Can you work these out from the model? Positions are in its coordinate system, mm. Face numbers are marked on the shaded views. A direction names the side the tool comes from. Round coordinates to 2 decimals unless told otherwise and drop trailing zeros. Loops run counter-clockwise (first coordinate to the right, second up) from the corner with the lowest first, then second, coordinate; pieces in that order, holes last.
from build123d import *

# Parameters (mm, degrees)
F1_DEPTH = 40
F2_R     = 19.99999
F3_F1_R  = 5
F3_F2_R  = 5
F4_R     = 16
F4_R_2   = 14
F5_DEPTH = 66.5


# Not quite as in the source:
# - a fillet or chamfer is up to 0.001 mm smaller than in the source, because OpenCascade refuses the exact size
# - ends of sketch curves that miss each other by under 0.0002 mm in the source are joined


with BuildPart() as f1:
    # F0 (on Top) → F1 (new body)
    with BuildSketch(Plane.XY):
        Polygon((-72.9024875954, 30), (-72.9024875954, 0), (-37.9024875954, 0), (-19.8747312181, 30), (17.0975124046, 30), (54.0697560273, 30), (72.0975124046, 0), (107.0975124046, 0), (107.0975124046, 30), (72.0975124046, 30), (54.0697560273, 60), (17.0975124046, 60), (-19.8747312181, 60), (-37.9024875954, 30), align=None)
    extrude(amount=F1_DEPTH)

    # F2 (radius 20 in the source; OpenCascade refuses exactly that, so slightly less here)
    f2_edges = [f1.edges().sort_by_distance(p)[0] for p in [
        (-72.902488, 15, 40),
        (-72.902488, 15, 0),
        (107.097512, 15, 40),
        (107.097512, 15, 0),
    ]]
    fillet(f2_edges, radius=F2_R)

    # F3: fillet of radius 5 on 16 edges, made by hand

    # F3_f1
    f3_f1_edges = [f1.edges().sort_by_distance(p)[0] for p in [
        (-19.8747312181, 30, 20),
        (54.0697560273, 30, 20),
        (72.0975124046, 30, 20),
        (-37.9024875954, 30, 20),
    ]]
    fillet(f3_f1_edges, radius=F3_F1_R)

    # F3_f2
    f3_f2_edges = [f1.edges().sort_by_distance(p)[0] for p in [
        (-37.9024875954, 0, 20),
        (72.0975124046, 0, 20),
        (54.0697560273, 60, 20),
        (-19.8747312181, 60, 20),
        (62.3551307083, 46.2123031159, 40),
        (17.0975124046, 60, 40),
        (-28.1601058991, 46.2123031159, 40),
        (63.8121377235, 13.7876968841, 40),
        (101.2396509572, 0, 5.8578614473),
        (-67.0446261481, 0, 5.8578614473),
        (17.0975124046, 30, 0),
        (17.0975124046, 60, 0),
        (-72.9024875954, 0, 20),
        (-45.4024925954, 0, 0),
        (-67.0446261481, 0, 34.1421385527),
        (-45.4024925954, 0, 40),
        (107.0975124046, 0, 20),
        (79.5975174046, 0, 0),
        (101.2396509572, 0, 34.1421385527),
        (79.5975174046, 0, 40),
        (-19.5080384845, 29.3518369019, 0),
        (53.7030632936, 29.3518369019, 0),
        (53.7030632936, 29.3518369019, 40),
        (-38.269180329, 30.6481630981, 40),
        (72.4642051382, 30.6481630981, 40),
    ]]
    fillet(f3_f2_edges, radius=F3_F2_R)

    # F4 (on face) → F5 (cut)
    with BuildSketch(Plane.XZ):
        with BuildLine():
            Line((-40.7311948659, 9.6144507468), (-40.7311948659, 30.3855492532))
            ThreePointArc((-40.7311948659, 30.3855492532), (-43.7377821689, 33.1151886927), (-47.3347232326, 35))
            Line((-47.3347232326, 35), (-52.9024975954, 35))
            ThreePointArc((-52.9024975954, 35), (-63.5090922422, 30.6066046467), (-67.9024875954, 20.00001))
            ThreePointArc((-67.9024875954, 20.00001), (-63.5090922422, 9.3933953533), (-52.9024975954, 5))
            Line((-52.9024975954, 5), (-47.3347232326, 5))
            ThreePointArc((-47.3347232326, 5), (-43.7377821689, 6.8848113073), (-40.7311948659, 9.6144507468))
        make_face()
        with Locations((87.0975124046, 20)):
            Circle(F4_R)
        with BuildLine():
            ThreePointArc((-40.7311948659, 9.6144507468), (-37.8901479431, 14.4655932419), (-36.9024875954, 20))
            ThreePointArc((-36.9024875954, 20), (-37.8901479431, 25.5344067581), (-40.7311948659, 30.3855492532))
            Line((-40.7311948659, 30.3855492532), (-40.7311948659, 9.6144507468))
        make_face()
        with Locations((17.0975124046, 20)):
            Circle(F4_R_2)
    extrude(amount=-F5_DEPTH, mode=Mode.SUBTRACT)


solid = f1.part
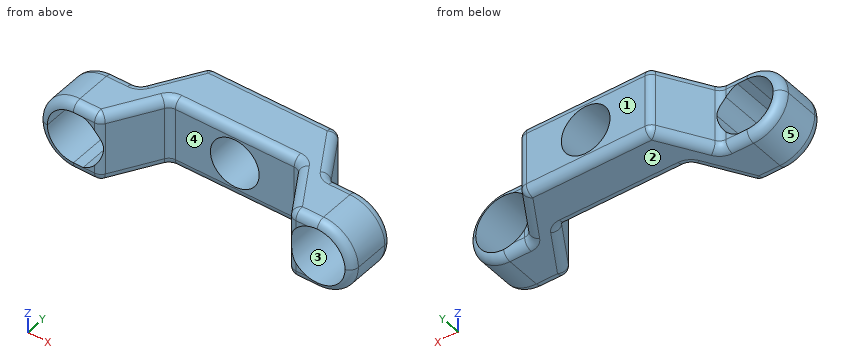
(1) If we section it at B-B, the plane y = 17: State how many separate pieces and enclosed holes the cut face has, then the cut area to 3 significant figures.
Worked answers:
separate pieces: 2
enclosed holes: 2
area: 1,700 mm2
(2) If we section it at A-A, the plane x = 46: List the corners of the cut face in (y, z) for me, then the cut area to 3 significant figures.
Worked answers:
outline: (30, 5) arc R5 ccw to (35, 0) - (55, 0) arc R5 ccw to (60, 5) - (60, 35) arc R5 ccw to (55, 40) - (35, 40) arc R5 ccw to (30, 35) - close
area: 1,180 mm2
(3) For the marked faces 4 and 5, which set-ups out of +Z, -Z, +X, -X, +Y, -Y let a thin tool reach every point of the face, with its end or its side?
Worked answers:
face 4: +Z, -Z, -Y
face 5: -Z, -X, +Y, -Y
(4) If I drill on line 1 (X direction, y = 15, z = 20); line 2 (X direction, y = 17, z = 20); line 3 (Y direction, x = 39.5, z = 6), over which ranges is the centre line in solid material (lowest first)?
Worked answers:
line 1: x = -72.9 to -67.9, -36.9 to -28.89, 63.08 to 71.1, 103.1 to 107.1
line 2: x = -72.9 to -67.9, -36.9 to -27.69, 61.88 to 71.1, 103.1 to 107.1
line 3: y = 30 to 60
(5) Will these pins go through, and if not, where does the flat tip stop? P1, Ø3.5, axis at x = 77, z = 32.5, coming from the +Y side; P2, Ø10, axis at y = 52, z = 23.5, coming from the +X side; P3, Ø3, axis at y = 10.5, z = 10.5, coming from the -X side; P4, Ø12, axis at y = 10, z = 15, coming from the -X side.
Worked answers:
P1: stops at y = 30
P2: stops at x = 61.88
P3: stops at x = -71.23
P4: stops at x = -72.9
(6) If we mould it in two halves opening along Z, with no side actions, what happens to the marked faces 1, 2 and 3? For each: released by +Z, released by -Z, zero draft, split by the parting line, or undercut.
Worked answers:
face 1: zero draft
face 2: released by -Z
face 3: undercut
